```python
from build123d import *

# Parameters (mm, degrees)
SKETCH3_R               = 1.778
BOSS_EXTRUDE2_DEPTH     = 38.1
CUT_EXTRUDE3_DEPTH      = 65.707715151
CUT_EXTRUDE3_DEPTH_BACK = 65.707715151
SKETCH11_W              = 22.86
SKETCH11_H              = 50.8
SKETCH8_R               = 1.778
CUT_EXTRUDE4_DEPTH      = 65.707715151


with BuildPart() as part:
    # Sketch3 → Boss-Extrude2 (new body)
    with BuildSketch(Plane.XY):
        with BuildLine():
            Line((12.7, -38.1), (25.4, -38.1))
            Line((25.4, -38.1), (25.4, -45.72))
            Line((25.4, -45.72), (-25.4, -45.72))
            Line((-25.4, -45.72), (-25.4, -38.1))
            Line((-25.4, -38.1), (-12.7, -38.1))
            Line((-12.7, -38.1), (-12.7, 0))
            ThreePointArc((-12.7, 0), (0, 12.7), (12.7, 0))
            Line((12.7, 0), (12.7, -38.1))
        make_face()
        with Locations(Location((0, 0, 0), (0, 0, 180))):
            Circle(SKETCH3_R, mode=Mode.SUBTRACT)
        with Locations(Location((0, -12.7, 0), (0, 0, 180))):
            Circle(SKETCH3_R, mode=Mode.SUBTRACT)
        with Locations(Location((0, -25.4, 0), (0, 0, 180))):
            Circle(SKETCH3_R, mode=Mode.SUBTRACT)
    extrude(amount=BOSS_EXTRUDE2_DEPTH)

    # Sketch11 → Cut-Extrude3 (cut, two sides: drawn at the far end of the back side and taken through both)
    with BuildSketch(Plane(origin=(0, 0, 0), x_dir=(0, 0, -1), z_dir=(1, 0, 0)).offset(-CUT_EXTRUDE3_DEPTH_BACK)):
        with Locations((-19.05, -12.7)):
            Rectangle(SKETCH11_W, SKETCH11_H)
    extrude(amount=CUT_EXTRUDE3_DEPTH + CUT_EXTRUDE3_DEPTH_BACK, mode=Mode.SUBTRACT)

    # Sketch8 → Cut-Extrude4 (cut, through all)
    with BuildSketch(Plane(origin=(0, 0, 0), x_dir=(1, 0, 0), z_dir=(0, 1, 0))):
        with Locations(Location((-17.78, -7.62, 0), (0, 0, 270))):
            Circle(SKETCH8_R)
        with Locations(Location((17.78, -7.62, 0), (0, 0, 270))):
            Circle(SKETCH8_R)
        with Locations(Location((17.78, -30.48, 0), (0, 0, 270))):
            Circle(SKETCH8_R)
        with Locations(Location((-17.78, -30.48, 0), (0, 0, 270))):
            Circle(SKETCH8_R)
    extrude(amount=-CUT_EXTRUDE4_DEPTH, mode=Mode.SUBTRACT)


solid = part.part
```
Here's how the part is built. I have some questions about the finished solid (model axes, mm). A direction names the side the tool comes from. Give positions to 0.01 mm unless a question says otherwise; leave off trailing zeros. Loops run counter-clockwise (first coordinate to the right, second up) from the corner with the lowest first, then second, coordinate; pieces in that order, holes last. Notation, with made-up numbers: (31, -14.75) -> (57, -14.75) arc R14 ccw to (57, -3.75) -> close; hole circle Ø11 at (39, 9). An arc over 180 degrees is marked (long way). Use one line per item in the form item = value. Start each with the question number.
1) Please list where these lines run through material, in increasing order: line 1 along Y through (x, z) = (0, 3.25); line 2 along Z through (x, y) = (6, -7); line 3 along X through (y, z) = (-25.4, 34.75).
2) Which directions (+Z, -Z, +X, -X, +Y, -Y) give clear straight access to the entire face, cutting with the end or side of a thin tool? Please do faces 5 (the face through (3, -13, 7.62)), 6 (the face through (0, -23, 38.1)), 7 (the face through (12.7, -19, 34)), 8 (the face through (-12.7, -19, 34)).
3) Thinking about a two-plate mould opening in X: for faces 1 (the face through (0.385, 1.736, 3.757)), 2 (the face through (-19.516, -41.857, 7.235)), 3 (the face through (-0.279, 12.697, 34.237)), 4 (the face through (25.4, -42, 19)), which applies, +X half, -X half, draft (parallel to the pull), parting line (faces both ways), or undercut?
4) For P1, Ø5, axis at x = 0, z = 14, coming from the +Y side; P2, Ø8.5, axis at y = -21.5, z = 3, coming from the -X side; P3, Ø8.5, axis at y = -19, z = 33, coming from the +X side, each with a flat end and sliding along its axis, tell me the tip position at first contact or that it passes through.
5) Imagine slicing it at B-B (y = -20). Please give me the cut outline in (x, z).
6) Imagine slicing it at D-D (y = 9.5). Please give me the cut outline in (x, z).
7) Imagine slicing it at A-A (x = 0). Count the separate pieces of the cut face and the enclosed holes in it, then the cut area to 3 significant figures.
8) Imagine slicing it at C-C (x = 17.78). Please give me the cut outline in (y, z), then the cut area to 3 significant figures.
Check values:
q1.line_1 = -45.72 to -27.18, -23.62 to -14.48, -10.92 to -1.78, 1.78 to 12.7
q1.line_2 = 0 to 7.62, 30.48 to 38.1
q1.line_3 = -12.7 to -1.78, 1.78 to 12.7
q2.face_5 = +X, -X, +Y
q2.face_6 = +Z, +X, -X, +Y, -Y
q2.face_7 = +Z, -Z, +X, +Y
q2.face_8 = +Z, -Z, -X, +Y
q3.face_1 = undercut
q3.face_2 = undercut
q3.face_3 = parting line
q3.face_4 = +X half
q4.P1 = -38.1
q4.P2 = -12.7
q4.P3 = 12.7
q5.outline = (-12.7, 0) -> (12.7, 0) -> (12.7, 7.62) -> (-12.7, 7.62) -> close; (-12.7, 30.48) -> (12.7, 30.48) -> (12.7, 38.1) -> (-12.7, 38.1) -> close
q6.outline = (-8.43, 0) -> (8.43, 0) -> (8.43, 7.62) -> (-8.43, 7.62) -> close; (-8.43, 30.48) -> (8.43, 30.48) -> (8.43, 38.1) -> (-8.43, 38.1) -> close
q7.separate_pieces = 7
q7.enclosed_holes = 0
q7.area = 902 mm^2
q8.outline = (-45.72, 0) -> (-38.1, 0) -> (-38.1, 5.84) -> (-45.72, 5.84) -> close; (-45.72, 9.4) -> (-38.1, 9.4) -> (-38.1, 28.7) -> (-45.72, 28.7) -> close; (-45.72, 32.26) -> (-38.1, 32.26) -> (-38.1, 38.1) -> (-45.72, 38.1) -> close
q8.area = 236 mm^2
